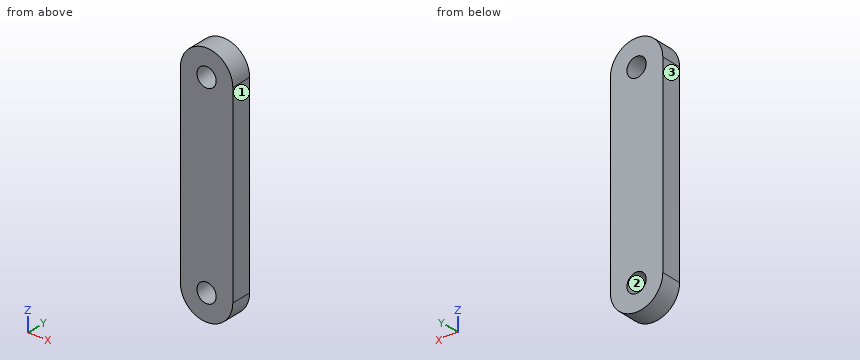
Autodesk Inventor part; units mm, degrees
ref_plane "Work Plane1" through (0, 0, -27.5) normal (0, 0, 1) x (1, 0, 0)
ref_plane "YZ Plane" through (0, 0, 0) normal (1, 0, 0) x (0, 1, 0)
ref_plane "XZ Plane" through (0, 0, 0) normal (0, 1, 0) x (-1, 0, 0)
sketch "Sketch1" plane through (0, 0, 0) normal (0, 1, 0) x (-1, 0, 0)
  circle A0 centre (0, 0) radius 2.75
  line L0 (0, 0) -> (0, -55) construction
  circle A1 centre (0, -55) radius 2.75
  line L1 (0, 0) -> (0, -55) construction
  line L2 (-7.5, 0) -> (-7.5, -55)
  line L3 (7.5, -55) -> (7.5, 0)
  arc A2 (7.5, 0) -> (-7.5, 0) centre (0, 0) ccw
  arc A3 (-7.5, -55) -> (7.5, -55) centre (0, -55) ccw
  point P0 (0, -27.5)
  dimension "d0" = 5.5
  dimension "d1" = 55
  dimension "d2" = 5.5
  dimension "d3" = 15
extrude "Extrusion1" add sketch "Sketch1" along normal blind 6
ref_plane "Work Plane1" through (0, 0, -27.5) normal (0, 0, 1) x (1, 0, 0)
properties part number "BaseTensionBracket" material "Aluminum 6061"
Could you check a few things on this model? Use its own coordinates, in mm. Face numbers are marked on the shaded views. Give positions to 0.01 mm unless a question says otherwise; leave off trailing zeros. Order: outer loops, then holes, each group sorted by start corner. A loop starts at its lowest first (then second) coordinate and runs counter-clockwise, first axis right, second up. Notation, with made-up numbers: (85, -11.75) - (120, -11.75) arc R24 ccw to (120, 7.25) - close; hole circle Ø11 at (63.5, -1.75). An arc over 180 degrees is marked (long way). Return JSON: item names as keys, results as strings. Group by question number.
Q1. Please list where these lines run through material, in increasing order: line 1 along Z through (x, y) = (0, 1.6); line 2 along Z through (x, y) = (1.75, 5.2); line 3 along X through (y, z) = (2.35, 4). Write a range as [from, to].
Q2. Suppose I cut it at B-B, the plane y = 1.5. Please give me the cut outline in (x, z), and give its area (3 significant figures).
Q3. Will these pins go through, and if not, where does the flat tip stop? pin 1 Ø1 at (x, y) = (-2.5, 4) entering from -Z; pin 2 Ø6.5 at (x, z) = (0, -55) entering from -Y; pin 3 Ø5 at (x, z) = (0, 0) entering from +Y; pin 4 Ø3 at (x, y) = (5, 3) entering from -Z.
Q4. Thinking about a two-plate mould opening in X: for the marked faces 1, 2 and 3, which applies, pulls with the +X half, pulls with the -X half, needs draft (parallel to the pull), parting line crosses it, or undercut?
Q5. Suppose I cut it at A-A, the plane x = 0. Please give me the cut outline in (y, z), and give its area (3 significant figures).
Resolved:
{
 "1": {"line 1": "z = [-62.5, -57.75], [-52.25, -2.75], [2.75, 7.5]", "line 2": "z = [-62.29, -57.12], [-52.88, -2.12], [2.12, 7.29]", "line 3": "x = [-6.34, 6.34]"},
 "2": {"outline": "(-7.5, -55) arc R7.5 ccw to (7.5, -55) - (7.5, 0) arc R7.5 ccw to (-7.5, 0) - close; hole circle Ø5.5 at (0, -55); hole circle Ø5.5 at (0, 0)", "area": "954 mm2"},
 "3": {"pin 1": "stops at z = -62.23", "pin 2": "stops at y = 0", "pin 3": "passes through", "pin 4": "stops at z = -61.63"},
 "4": {"face 1": "pulls with the +X half", "face 2": "undercut", "face 3": "pulls with the -X half"},
 "5": {"outline": "(0, -62.5) - (6, -62.5) - (6, -57.75) - (0, -57.75) - close; (0, -52.25) - (6, -52.25) - (6, -2.75) - (0, -2.75) - close; (0, 2.75) - (6, 2.75) - (6, 7.5) - (0, 7.5) - close", "area": "354 mm2"}
}
